from build123d import *

# Parameters (mm, degrees)
SKETCH1_W           = 82
SKETCH1_H           = 11
BOSS_EXTRUDE1_DEPTH = 50
SKETCH2_R           = 1.6
CUT_EXTRUDE1_DEPTH  = 10
SKETCH3_R           = 1.6
CUT_EXTRUDE2_DEPTH  = 10
SKETCH4_R           = 1.6
CUT_EXTRUDE3_DEPTH  = 15


with BuildPart() as part:
    # Sketch1 → Boss-Extrude1 (new body)
    with BuildSketch(Plane.XY):
        with Locations((-41, 5.5)):
            Rectangle(SKETCH1_W, SKETCH1_H)
    extrude(amount=BOSS_EXTRUDE1_DEPTH)

    # Sketch2 → Cut-Extrude1 (cut)
    with BuildSketch(Plane(origin=(0, 0, 0), x_dir=(0, 0, -1), z_dir=(1, 0, 0))):
        with Locations((-5.6, 5.5)):
            Circle(SKETCH2_R)
    extrude(amount=-CUT_EXTRUDE1_DEPTH, mode=Mode.SUBTRACT)

    # Sketch3 → Cut-Extrude2 (cut)
    with BuildSketch(Plane.ZY.offset(82)):
        with Locations((5.6, 5.5)):
            Circle(SKETCH3_R)
    extrude(amount=-CUT_EXTRUDE2_DEPTH, mode=Mode.SUBTRACT)

    # Sketch4 → Cut-Extrude3 (cut)
    with BuildSketch(Plane.XY.offset(50)):
        with Locations((-76, 5.5)):
            Circle(SKETCH4_R)
        with Locations((-6, 5.5)):
            Circle(SKETCH4_R)
    extrude(amount=-CUT_EXTRUDE3_DEPTH, mode=Mode.SUBTRACT)


solid = part.part
Read the model definition and answer for the solid it produces. Units are mm, in the model's axes. A direction names the side the tool comes from. Give positions to 0.01 mm unless a question says otherwise; leave off trailing zeros. Write each loop counter-clockwise with the first axis right and the second up, starting at its lowest first coordinate (ties: lowest second). Pieces come first, ordered by that corner, then holes. Notation, with made-up numbers: (-34, 82) -> (-24, 82) arc R29 ccw to (-24, 102) -> close; hole circle Ø6 at (14, -11.75). An arc over 180 degrees is marked (long way). Answer as a JSON object with one key per item and string values. Group by question number.
1) Find section A-A (x = -6). Write down the section's boundary in (y, z), and give its area (3 significant figures).
2) A tool of negligible diameter and unlimited length cuts with its end or side. For faces 1 (the cylindrical face through (-77.07, 4.53, 4.33)), 2 (the flat face through (-6, 6, 35)), 3 (the flat face through (0, 5, 25)), 4 (the cylindrical face through (-4.93, 4.53, 6.87)), from which of +Z, -Z, +X, -X, +Y, -Y can it reach the whole face along a straight path? Write none if from no direction.
3) Consider L1, parallel to Y at x = -76, z = 44; L2, parallel to Y at x = -72.5, z = 5. Determine where each line is inside the solid, lowest interval first. Write a range as from..to.
4) Each of these flat-tipped pins is pushed along its axis until it touches: P1, Ø1, axis at x = -6, y = 6, coming from the +Z side; P2, Ø1.6, axis at y = 6, z = 5.5, coming from the -X side. Where does it stop, or does it pass through?
5) Find section C-C (y = 5.5). Write down the section's boundary in (x, z).
6) The mould has two halves that part along X. Classify faces 5 (the flat face through (-82, 5, 25)), 6 (the flat face through (-42, 11, 25)), 7 (the cylindrical face through (-5.26, 4.08, 42.6)): +X half, -X half, draft (parallel to the pull), parting line (faces both ways), or undercut.
7) Find section B-B (z = 41.5). Write down the section's boundary in (x, y).
Values follow:
{
 "1": {"outline": "(0, 0) -> (11, 0) -> (11, 50) -> (7.1, 50) -> (7.1, 35) -> (3.9, 35) -> (3.9, 50) -> (0, 50) -> close; hole circle Ø3.2 at (5.5, 5.6)", "area": "494 mm2"},
 "2": {"face 1": "-X", "face 2": "+Z", "face 3": "+Z, -Z, +X, +Y, -Y", "face 4": "+X"},
 "3": {"L1": "y = 0..3.9, 7.1..11", "L2": "y = 0..4.02, 6.98..11"},
 "4": {"P1": "stops at z = 35", "P2": "stops at x = -72"},
 "5": {"outline": "(-82, 0) -> (0, 0) -> (0, 4) -> (-10, 4) -> (-10, 7.2) -> (0, 7.2) -> (0, 50) -> (-4.4, 50) -> (-4.4, 35) -> (-7.6, 35) -> (-7.6, 50) -> (-74.4, 50) -> (-74.4, 35) -> (-77.6, 35) -> (-77.6, 50) -> (-82, 50) -> (-82, 7.2) -> (-72, 7.2) -> (-72, 4) -> (-82, 4) -> close"},
 "6": {"face 5": "-X half", "face 6": "draft", "face 7": "undercut"},
 "7": {"outline": "(-82, 0) -> (0, 0) -> (0, 11) -> (-82, 11) -> close; hole circle Ø3.2 at (-76, 5.5); hole circle Ø3.2 at (-6, 5.5)"}
}
